Input: part model. Units: mm. Frame: model coordinates. Face numbers are marked on the shaded views. A direction names the side the tool comes from. Coordinates: 2 decimals unless noted, no trailing zeros. Write each loop counter-clockwise with the first axis right and the second up, starting at its lowest first coordinate (ties: lowest second). Pieces come first, ordered by that corner, then holes.
1) Section query A-A (y = 0). Output: boundary loops of the cut face in (x, z).
2) Section query C-C (z = 1.8). Output: boundary loops of the cut face in (x, y), then the cut area to 3 significant figures.
3) Set-up query: the marked faces 4 and 5. Return all of +Z, -Z, +X, -X, +Y, -Y with unobstructed straight access to the full face (end or side cutting, diameter ignored); none if empty.
4) Section query B-B (x = 0). Output: boundary loops of the cut face in (y, z).
5) Line query: L1, parallel to X at y = -6.5, z = 2.5; L2, parallel to Y at x = 8.5, z = 4; L3, parallel to Y at x = 6, z = 2.85. Output: solid intervals per line, ascending.
6) Section query D-D (y = -17.5). Output: boundary loops of the cut face in (x, z).
7) Pin query (flat end, axial travel): pin 1 Ø1.5 at (y, z) = (20.5, 3.5) entering from -X; pin 2 Ø1.5 at (x, z) = (23, 2) entering from -Y; pin 3 Ø1.5 at (y, z) = (18.5, 3) entering from +X; pin 4 Ø9 at (x, y) = (0, 0) entering from -Z. Return the tip coordinate at first contact, or that it passes through.
8) Draft query along X for the marked faces 1, 2 and 3. Return one class per face: pulls with the +X half, pulls with the -X half, needs draft (parallel to the pull), parting line crosses it, or undercut.
from build123d import *

# Parameters (mm, degrees)
SKETCH1_R           = 30
SKETCH1_R_2         = 5
BOSS_EXTRUDE1_DEPTH = 5


with BuildPart() as part:
    # Sketch1 → Boss-Extrude1 (new body)
    with BuildSketch(Plane.XY):
        Circle(SKETCH1_R)
        Circle(SKETCH1_R_2, mode=Mode.SUBTRACT)
        with BuildLine():
            Line((-5, 24.494897428), (-5, 8.660254038))
            ThreePointArc((-5, 8.660254038), (-10, 0), (-5, -8.660254038))
            Line((-5, -8.660254038), (-5, -24.494897428))
            ThreePointArc((-5, -24.494897428), (-25, 0), (-5, 24.494897428))
        make_face(mode=Mode.SUBTRACT)
        with BuildLine():
            Line((5, 24.494897428), (5, 8.660254038))
            ThreePointArc((5, 8.660254038), (10, 0), (5, -8.660254038))
            Line((5, -8.660254038), (5, -24.494897428))
            ThreePointArc((5, -24.494897428), (25, 0), (5, 24.494897428))
        make_face(mode=Mode.SUBTRACT)
    extrude(amount=BOSS_EXTRUDE1_DEPTH)


solid = part.part
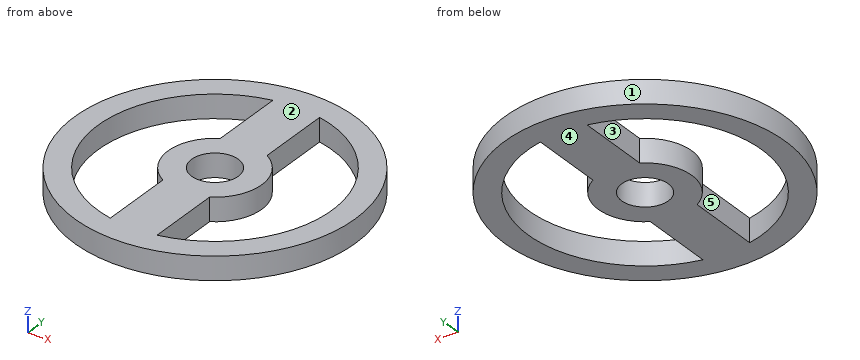
Answer:
1. outline: (-30, 0) - (-25, 0) - (-25, 5) - (-30, 5) - close; (-10, 0) - (-5, 0) - (-5, 5) - (-10, 5) - close; (5, 0) - (10, 0) - (10, 5) - (5, 5) - close; (25, 0) - (30, 0) - (30, 5) - (25, 5) - close
2. outline: circle Ø60 at (0, 0); hole (-5, -24.49) - (-5, -8.66) arc R10 cw to (-5, 8.66) - (-5, 24.49) arc R25 ccw to start; hole circle Ø10 at (0, 0); hole (5, -24.49) arc R25 ccw to (5, 24.49) - (5, 8.66) arc R10 cw to (5, -8.66) - close
2. area: 1,400 mm2
3. face 4: -Z, +X, -X, +Y, -Y
3. face 5: +Z, -Z
4. outline: (-30, 0) - (-5, 0) - (-5, 5) - (-30, 5) - close; (5, 0) - (30, 0) - (30, 5) - (5, 5) - close
5. L1: x = -29.29 to -24.14, -7.6 to 7.6, 24.14 to 29.29
5. L2: y = -28.77 to -23.51, -5.27 to 5.27, 23.51 to 28.77
5. L3: y = -29.39 to -24.27, -8 to 8, 24.27 to 29.39
6. outline: (-24.37, 0) - (-17.85, 0) - (-17.85, 5) - (-24.37, 5) - close; (-5, 0) - (5, 0) - (5, 5) - (-5, 5) - close; (17.85, 0) - (24.37, 0) - (24.37, 5) - (17.85, 5) - close
7. pin 1: stops at x = -22.58
7. pin 2: stops at y = -20.12
7. pin 3: stops at x = 24.19
7. pin 4: passes through
8. face 1: parting line crosses it
8. face 2: needs draft
8. face 3: undercut
